from build123d import *

# Parameters (mm, degrees)
BOSS_EXTRUDE1_DEPTH = 8
SKETCH2_W           = 2.1
SKETCH2_H           = 6
CUT_EXTRUDE1_DEPTH  = 8
CUT_EXTRUDE2_DEPTH  = 6


with BuildPart() as part:
    # Sketch1 → Boss-Extrude1 (new body)
    with BuildSketch(Plane.XY):
        Polygon((0, 9), (0, 12), (10, 12), (10, 0), (0, 0), (0, 3), (7.85, 3), (7.85, 9), align=None)
    extrude(amount=BOSS_EXTRUDE1_DEPTH)

    # Sketch2 → Cut-Extrude1 (cut)
    with BuildSketch(Plane(origin=(10, 0, 0), x_dir=(0, 0, -1), z_dir=(1, 0, 0))):
        with Locations((-6.95, 6)):
            Rectangle(SKETCH2_W, SKETCH2_H)
        with Locations((-1.05, 6)):
            Rectangle(SKETCH2_W, SKETCH2_H)
    extrude(amount=-CUT_EXTRUDE1_DEPTH, mode=Mode.SUBTRACT)

    # Sketch3 → Cut-Extrude2 (cut)
    with BuildSketch(Plane(origin=(0, 3, 0), x_dir=(1, 0, 0), z_dir=(0, 1, 0))):
        with BuildLine():
            Line((10, -2.1), (8.925, -2.1))
            ThreePointArc((8.925, -2.1), (9.487750142, -2.185251456), (10, -2.433355497))
            Line((10, -2.433355497), (10, -2.1))
        make_face()
        with BuildLine():
            Line((8.925, -2.1), (7.85, -2.1))
            Line((7.85, -2.1), (7.85, -2.433355497))
            ThreePointArc((7.85, -2.433355497), (8.362249858, -2.185251456), (8.925, -2.1))
        make_face()
        with BuildLine():
            Line((7.85, -5.566644503), (7.85, -5.9))
            Line((7.85, -5.9), (8.925, -5.9))
            ThreePointArc((8.925, -5.9), (8.362249858, -5.814748544), (7.85, -5.566644503))
        make_face()
        with BuildLine():
            ThreePointArc((10, -5.566644503), (9.487750142, -5.814748544), (8.925, -5.9))
            Line((8.925, -5.9), (10, -5.9))
            Line((10, -5.9), (10, -5.566644503))
        make_face()
    extrude(amount=CUT_EXTRUDE2_DEPTH, mode=Mode.SUBTRACT)


solid = part.part
Check sheet for the modelled part. Datum: model origin and axes. Units: mm. A direction names the side the tool comes from. Round coordinates to 2 decimals unless told otherwise and drop trailing zeros. Order: outer loops, then holes, each group sorted by start corner. A loop starts at its lowest first (then second) coordinate and runs counter-clockwise, first axis right, second up.
(1) Access from +Z, -Z, +X, -X, +Y, -Y to the whole of each face (thin tool, end or side, straight path). Record for faces 4 (the flat face through (5, 11, 0)), 5 (the flat face through (7.85, 6, 4)).
(2) Cross-section at B-B, the plane z = 3.75. Enter the section's corners in (x, y), and give its area (3 significant figures).
(3) Cross-section at D-D, the plane x = 8. Enter the section's corners in (y, z), and give its area (3 significant figures).
(4) Scan lines: probe 1 along Y at (x, z) = (5, 4); probe 2 along X at (y, z) = (6.5, 4.5); probe 3 along Z at (x, y) = (8, 4). Record each from-to range of solid material in increasing order.
(5) Cross-section at A-A, the plane x = 2. Enter the section's corners in (y, z), and give its area (3 significant figures).
(6) Go/stop test with a flat-tipped pin: P1, Ø1.6, axis at y = 5, z = 3.5, coming from the -X side. Record where the tip stops, or that it passes through.
(7) Cross-section at C-C, the plane y = 5.5. Enter the section's corners in (x, z) (3 decimals), and give its area (3 significant figures).
(8) Draft check along Y on faces 1 (the flat face through (10, 6, 4)), 2 (the flat face through (5, 3, 4)), 3 (the flat face through (5, 0, 4)). Enter one of: pulls with the +Y half, pulls with the -Y half, needs draft (parallel to the pull), parting line crosses it, or undercut.
Check sheet entries:
1. face 4: -Z, +X, -X, +Y, -Y
1. face 5: +Z, -Z, -X
2. outline: (0, 0) - (10, 0) - (10, 12) - (0, 12) - (0, 9) - (7.85, 9) - (7.85, 3) - (0, 3) - close
2. area: 72.9 mm2
3. outline: (0, 0) - (3, 0) - (3, 2.34) - (9, 2.34) - (9, 0) - (12, 0) - (12, 8) - (9, 8) - (9, 5.66) - (3, 5.66) - (3, 8) - (0, 8) - close
3. area: 67.9 mm2
4. probe 1: y = 0 to 3, 9 to 12
4. probe 2: x = 7.85 to 10
4. probe 3: z = 2.34 to 5.66
5. outline: (0, 0) - (3, 0) - (3, 8) - (0, 8) - close; (9, 0) - (12, 0) - (12, 8) - (9, 8) - close
5. area: 48.0 mm2
6. P1: stops at x = 7.85
7. outline: (7.85, 2.433) arc R1.9 ccw to (10, 2.433) - (10, 5.567) arc R1.9 ccw to (7.85, 5.567) - close
7. area: 7.71 mm2
8. face 1: needs draft
8. face 2: undercut
8. face 3: pulls with the -Y half
